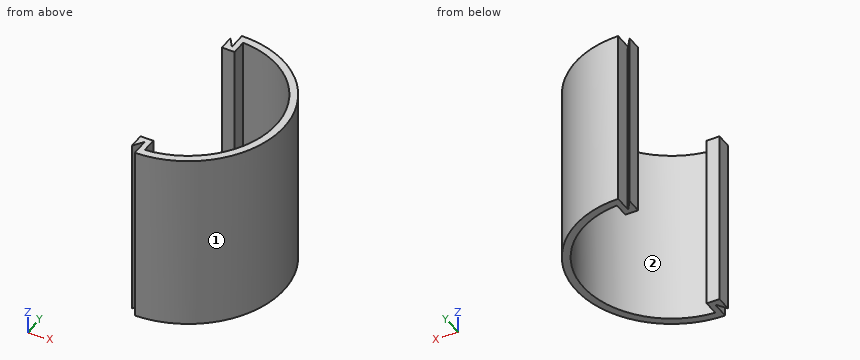
Autodesk Fusion 360 part; units mm, degrees
sketch "Sketch4" plane through (0, 0, 0) normal (0, 0, 1) x (1, 0, 0)
  line L0 (0, 37.5) -> (0, -37.5)
  line L1 (0, 0) -> (37.5, 0)
  arc A0 (0, -34.5) -> (0, 34.5) centre (0, 0) ccw
  arc A1 (0, -37.5) -> (0, 37.5) centre (0, 0) ccw
  line L2 (0, 37.5) -> (-2.5, 37.5) construction
  line L3 (0, 34.5) -> (0, 30.5)
  line L4 (0, 30.5) -> (-2.8008, 34.5)
  line L5 (-2.8008, 34.5) -> (-2.8008, 28.5)
  line L6 (-2.8008, 28.5) -> (2.1992, 28.5)
  line L7 (2.1992, 28.5) -> (2.1992, 34.4298)
  line L8 (2.1992, -28.5) -> (2.1992, -34.4298)
  line L9 (0, -34.5) -> (0, -30.5)
  line L10 (0, -30.5) -> (-2.8008, -34.5)
  line L11 (-2.8008, -34.5) -> (-2.8008, -28.5)
  line L12 (-2.8008, -28.5) -> (2.1992, -28.5)
  dimension "d10" = 75
  dimension "d20" = 4
  dimension "d21" = 35
  dimension "d23" = 5
  dimension "d29" = 2
  dimension "d30" = 6
  dimension "d36" = 3
extrude "Extrude6" add sketch "Sketch4" along normal blind 70 contours L0 L1 A0 A1 | L0 A0 L3 L6 L7 | L0 L1 A0 A1 | L0 L4 L5 L6 | L0 A0 L8 L9 L12 | L0 L10 L11 L12 makes body 1
sketch "Sketch6" plane through (0, 0, 70) normal (0, 0, 1) x (-1, 0, 0)
  arc A0 (0, 37.5) -> (0, -37.5) centre (0, 0) ccw
  line L0 (0, 30.5) -> (0, 37.5)
  line L1 (0, -30.5) -> (2.8008, -34.5)
  line L2 (2.8008, -34.5) -> (2.8008, -28.5)
  line L3 (2.8008, -28.5) -> (-2.1992, -28.5)
  line L4 (0, 37.5) -> (0, -28.5)
  line L5 (0, -28.5) -> (2.8008, -28.5)
  line L6 (0, -30.5) -> (0, -28.5)
  line L7 (2.8008, -28.5) -> (2.8008, -34.5)
  line L8 (-2.1992, -31.9243) -> (-2.1992, -26)
  line L9 (-2.1992, -31.9243) -> (0, -31.9243)
  line L10 (-2.1992, -28.5) -> (-2.1992, -34.4298)
  arc A1 (-2.1992, 34.4298) -> (-2.1992, -34.4298) centre (0, 0) ccw
  line L11 (-2.1992, 34.4298) -> (-2.1992, 28.5)
  line L12 (-2.1992, 28.5) -> (2.8008, 28.5)
  line L13 (2.8008, 28.5) -> (2.8008, 34.5)
  line L14 (2.8008, 34.5) -> (0, 30.5)
  line L15 (0, -37.5) -> (0, -30.5)
  arc A2 (2.7253, -34.3922) -> (2.8008, -34.3861) centre (0, 0) ccw
  arc A3 (2.8008, 34.3861) -> (2.7253, 34.3922) centre (0, 0) ccw
  arc A4 (0, 34.5) -> (-2.1992, 34.4298) centre (0, 0) ccw
  arc A5 (-2.1992, -34.4298) -> (0, -34.5) centre (0, 0) ccw
extrude "Extrude7" cut sketch "Sketch6" against normal blind 1 contours L0 L4 L11 L12 A4 | L9 L10 L15 A5 | L4 L12 L13 L14 A3 | L3 L6 L8 L9 L10 L15 | L13 L14 A3 | L1 L2 L3 L5 L6 L7 A2 | L1 L2 L7 A2 bodies 1
mirror "Mirror2" about plane through (0, 0, 0) normal (0, 1, 0) of "Extrude7"
sketch "Sketch7" plane through (0, 0, 69) normal (0, 0, 1) x (-1, 0, 0)
  line L0 (2.8008, -34.5) -> (2.8008, -28.5)
  line L1 (2.8008, -28.5) -> (-2.1992, -28.5)
  line L2 (2.8008, -34.5) -> (2.8008, -28.5)
  line L3 (0, -30.5) -> (2.8008, -34.5)
  line L4 (0, -30.5) -> (2.8008, -34.5)
  line L5 (2.7008, -28.5) -> (2.7008, -34.1828)
  line L6 (2.7008, -34.1828) -> (0, -30.3257)
  line L7 (0, -30.5) -> (0, -30.3257)
  arc A0 (-2.1992, -34.4298) -> (0, -34.5) centre (0, 0) ccw
  dimension "d37" = 0.1
  dimension "d38" = 0.1
extrude "Extrude8" cut sketch "Sketch7" against normal blind 70 bodies 1
mirror "Mirror3" about plane through (0, 0, 0) normal (0, 1, 0) of "Extrude6", "Extrude7", "Extrude8", "Mirror2" makes body 2
fillet "Fillet1" radius 0.2 4 edges at (-2.7008, 34.1828, 34.5) (0, 30.3257, 34.5) (-2.7008, -34.1828, 34.5) (0, -30.3257, 34.5) on bodies 1 2
combine "Combine1" operation add target body 2 tool bodies 1
Source: CAD feature listing. Evaluate the final solid. Frame: model axes, mm. Face numbers are marked on the shaded views. Give positions to 0.01 mm unless a question says otherwise; leave off trailing zeros. Loops run counter-clockwise (first coordinate to the right, second up) from the corner with the lowest first, then second, coordinate; pieces in that order, holes last. Notation, with made-up numbers: M 39.25,-36 L 92.25,-36 A17 ccw 92.25,-7 Z; hole C 79.25,76 d4. An arc over 180 degrees is marked long. Put each result on its own line as item: value.
Q1. Pin query (flat end, axial travel): P1, Ø2, axis at x = 31, z = 7.5, coming from the -Y side; P2, Ø5, axis at x = 17, z = 33.5, coming from the +Y side; P3, Ø6, axis at y = -19, z = 16, coming from the +X side. Return the tip coordinate at first contact, or that it passes through.
Response values:
P1: stops at y = -22.5
P2: stops at y = 34.58
P3: stops at x = 33.92
Q2. Line query: probe 1 along Y at (x, z) = (6, 6.5); probe 2 along X at (y, z) = (-29, 6); probe 3 along Y at (x, z) = (10, 5). Output: solid intervals per line, ascending. Write a range as [from, to].
Response values:
probe 1: y = [-37.02, -33.97], [33.97, 37.02]
probe 2: x = [-2.8, 2.2], [18.69, 23.77]
probe 3: y = [-36.14, -33.02], [33.02, 36.14]
Q3. Section D-D (y = 0). Return the cut outline in (x, z), and give its area (3 significant figures).
Response values:
outline: M 34.5,0 L 37.5,0 L 37.5,70 L 34.5,70 Z
area: 210 mm²
Q4. Section B-B (z = 10). Return the cut outline in (x, y).
Response values:
outline: M -2.8,-34.5 L -0.18,-30.76 A0.2 cw 0,-30.96 L 0,-37.5 A37.5 ccw 0,37.5 L 0,30.96 A0.2 cw -0.18,30.76 L -2.8,34.5 L -2.8,28.5 L 2.2,28.5 L 2.2,34.43 A34.5 cw 2.2,-34.43 L 2.2,-28.5 L -2.8,-28.5 Z
Q5. Section A-A (x = 4.5). Return the cut outline in (y, z), and give its area (3 significant figures).
Response values:
outline: M -37.23,0 L -34.21,0 L -34.21,70 L -37.23,70 Z; M 34.21,0 L 37.23,0 L 37.23,70 L 34.21,70 Z
area: 423 mm²
Q6. Section C-C (y = 33.5). Return the cut outline in (x, z), and give its area (3 significant figures).
Response values:
outline: M -2.8,0 L -2.1,0 L -2.1,70 L -2.8,70 Z; M 0,0 L 2.2,0 L 2.2,70 L 0,70 Z; M 8.25,0 L 16.85,0 L 16.85,70 L 8.25,70 Z
area: 805 mm²
Q7. Mould query, pull axis X, two halves, no side actions, for the marked faces 1 and 2. Classes: released by +X, released by -X, zero draft, split by the parting line, or undercut.
Response values:
face 1: released by +X
face 2: undercut
